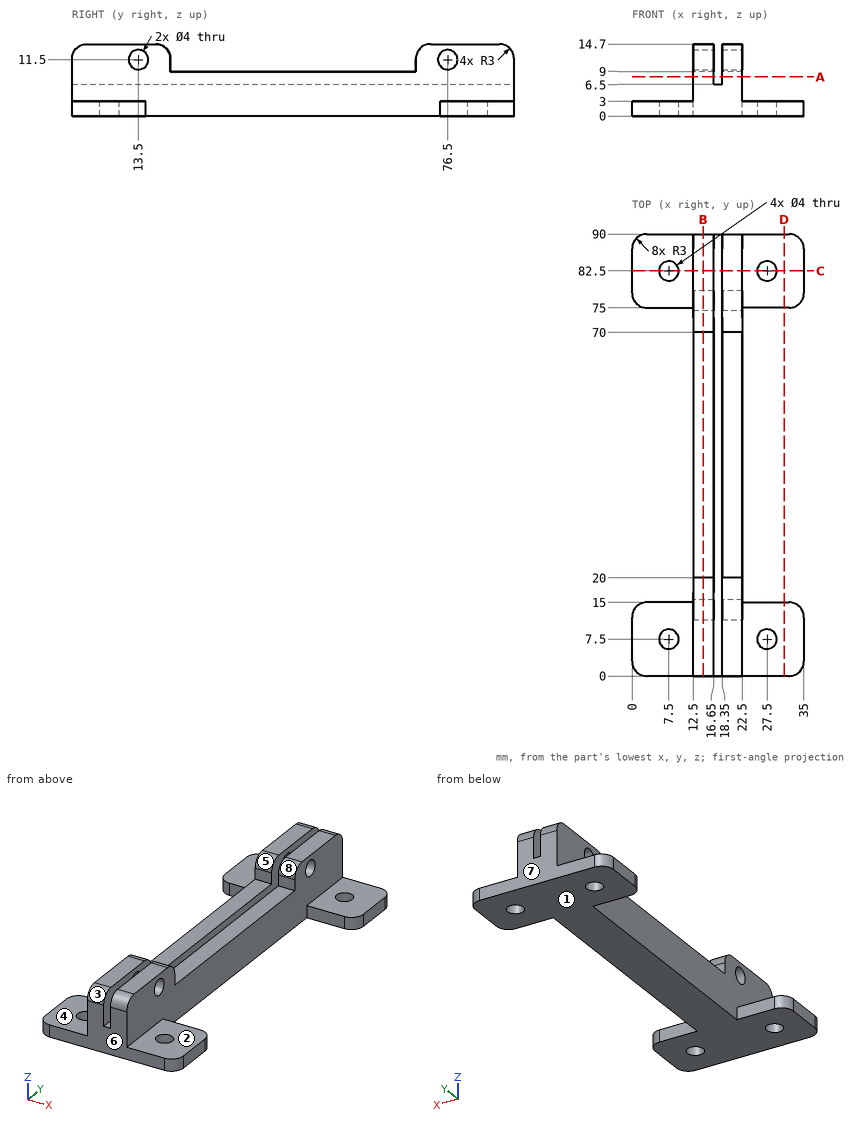
Could you check a few things on this drawing? It's one solid part, dimensions in mm from its lowest x, y, z. A direction names the side the tool comes from. Coordinates: 2 decimals unless noted, no trailing zeros. Write each loop counter-clockwise with the first axis right and the second up, starting at its lowest first coordinate (ties: lowest second). Pieces come first, ordered by that corner, then holes.
Q1. If we mould it in two halves opening along Y, with no side actions, what happens to the marked faces 6, 7 and 8? For each: +Y half, -Y half, draft (parallel to the pull), parting line (faces both ways), or undercut.
Results found:
face 6: -Y half
face 7: +Y half
face 8: undercut
Q2. Please list where these lines run through material, in increasing order: L1, parallel to X at y = 82.5, z = 1.3; L2, parallel to Y at x = 7.5, z = 2.1; L3, parallel to Z at x = 13.7, y = 76.5.
Results found:
L1: x = 0 to 5.5, 9.5 to 25.5, 29.5 to 35
L2: y = 0 to 5.5, 9.5 to 15, 75 to 80.5, 84.5 to 90
L3: z = 0 to 9.5, 13.5 to 14.7
Q3. Which directions (+Z, -Z, +X, -X, +Y, -Y) give clear straight access to the entire face, cutting with the end or side of a thin tool? Please do the marked faces 1, 2, 3, 4 and 5.
Results found:
face 1: -Z, +X, -X, +Y, -Y
face 2: +Z, +X, +Y, -Y
face 3: +Z, +X, -X, -Y
face 4: +Z, -X, +Y, -Y
face 5: +Z, +X, -X
Q4. Imagine slicing it at A-A, the plane z = 8. List the corners of the cut face in (x, y) for me.
Results found:
outline: (12.5, 0) - (16.65, 0) - (16.65, 90) - (12.5, 90) - close; (18.35, 0) - (22.5, 0) - (22.5, 90) - (18.35, 90) - close
Q5. Imagine slicing it at B-B, the plane x = 14.5. List the corners of the cut face in (y, z) for me.
Results found:
outline: (0, 0) - (90, 0) - (90, 11.7) arc R3 ccw to (87, 14.7) - (73, 14.7) arc R3 ccw to (70, 11.7) - (70, 9) - (20, 9) - (20, 11.7) arc R3 ccw to (17, 14.7) - (3, 14.7) arc R3 ccw to (0, 11.7) - close; hole circle Ø4 at (13.5, 11.5); hole circle Ø4 at (76.5, 11.5)
Q6. Imagine slicing it at D-D, the plane x = 31. List the corners of the cut face in (y, z) for me, plus the area to 3 significant figures.
Results found:
outline: (0, 0) - (15, 0) - (15, 3) - (0, 3) - close; (75, 0) - (90, 0) - (90, 3) - (75, 3) - close
area: 90.0 mm2
Q7. Imagine slicing it at C-C, the plane y = 82.5. List the corners of the cut face in (x, z) for me.
Results found:
outline: (0, 0) - (5.5, 0) - (5.5, 3) - (0, 3) - close; (9.5, 0) - (25.5, 0) - (25.5, 3) - (22.5, 3) - (22.5, 14.7) - (18.35, 14.7) - (18.35, 6.5) - (16.65, 6.5) - (16.65, 14.7) - (12.5, 14.7) - (12.5, 3) - (9.5, 3) - close; (29.5, 0) - (35, 0) - (35, 3) - (29.5, 3) - close
Q8. For P1, Ø0.9, axis at x = 17.5, y = 54, coming from the +Z side; P2, Ø6, axis at x = 4.5, y = 79, coming from the +Z side; P3, Ø3, axis at x = 20.5, z = 2.5, coming from the -Y side; P4, Ø2, axis at y = 30, z = 6, coming from the -X side, each with a flat end and sliding along its axis, tell me the tip position at first contact or that it passes through.
Results found:
P1: stops at z = 6.5
P2: stops at z = 3
P3: stops at y = 0
P4: stops at x = 12.5
